```python
from build123d import *
from build123d.topology import SkipClean

# Parameters (mm, degrees)
ESBO_O1_R                = 2
RESSALTO_EXTRUS_O1_DEPTH = 19
CORTE_EXTRUS_O1_DEPTH    = 18
ESBO_O3_R                = 2.5
RESSALTO_EXTRUS_O2_DEPTH = 7


with BuildPart() as part:
    # Esboço1 → Ressalto-extrusão1 (new body)
    with BuildSketch(Plane.XY):
        with BuildLine():
            Line((19, 3.5), (13.555441712, 3.5))
            ThreePointArc((13.555441712, 3.5), (0, 14), (-13.555441712, 3.5))
            Line((-13.555441712, 3.5), (-19, 3.5))
            ThreePointArc((-19, 3.5), (-22.5, 0), (-19, -3.5))
            Line((-19, -3.5), (-13.555441712, -3.5))
            ThreePointArc((-13.555441712, -3.5), (-11.320120282, -8.237407166), (-7.5, -11.821590418))
            Line((-7.5, -11.821590418), (-7.5, -14))
            Line((-7.5, -14), (-7.5, -17))
            Line((-7.5, -17), (7.5, -17))
            Line((7.5, -17), (7.5, -14))
            Line((7.5, -14), (7.5, -11.821590418))
            ThreePointArc((7.5, -11.821590418), (11.320120282, -8.237407166), (13.555441712, -3.5))
            Line((13.555441712, -3.5), (19, -3.5))
            ThreePointArc((19, -3.5), (22.5, 0), (19, 3.5))
        make_face()
        with Locations((19, 0)):
            Circle(ESBO_O1_R, mode=Mode.SUBTRACT)
        with Locations(Location((-19, 0, 0), (0, 0, 180))):
            Circle(ESBO_O1_R, mode=Mode.SUBTRACT)
    extrude(amount=RESSALTO_EXTRUS_O1_DEPTH)

    # Esboço2 → Corte-extrusão1 (cut)
    with SkipClean():  # the faces are left unmerged after this step: merging them gives an invalid solid
        with BuildSketch(Plane(origin=(0, 0, 0), x_dir=(-1, 0, 0), z_dir=(0, 0, -1))):
            with BuildLine():
                Line((13.555441712, 3.5), (23.80699558, 3.5))
                Line((23.80699558, 3.5), (23.80699558, -3.5))
                Line((23.80699558, -3.5), (13.555441712, -3.5))
                ThreePointArc((13.555441712, -3.5), (14, 0), (13.555441712, 3.5))
            make_face()
            with BuildLine():
                Line((-13.555441712, 3.5), (-24.760546325, 3.5))
                Line((-24.760546325, 3.5), (-24.760546325, -3.5))
                Line((-24.760546325, -3.5), (-13.555441712, -3.5))
                ThreePointArc((-13.555441712, -3.5), (-14, 0), (-13.555441712, 3.5))
            make_face()
        extrude(amount=-CORTE_EXTRUS_O1_DEPTH, mode=Mode.SUBTRACT)

    # Esboço3 → Ressalto-extrusão2 (add)
    with SkipClean():  # the faces are left unmerged after this step: merging them gives an invalid solid
        with BuildSketch(Plane.XY.offset(19)):
            with Locations((0, 6.5)):
                Circle(ESBO_O3_R)
        extrude(amount=RESSALTO_EXTRUS_O2_DEPTH)


solid = part.part
```
Geometry: final body of the model. Coordinates: model frame, mm. A direction names the side the tool comes from. Coordinates: 2 decimals unless noted, no trailing zeros. Loops run counter-clockwise (first coordinate to the right, second up) from the corner with the lowest first, then second, coordinate; pieces in that order, holes last. Notation, with made-up numbers: (64, 6) -> (91, 6) arc R15 cw to (91, 33) -> close; hole circle Ø6 at (-37.5, 65). An arc over 180 degrees is marked (long way). Use a Markdown table: item, result. Add a question column.
(1) Section query D-D, the plane x = 18. Return loops of the section in (y, z), plus the area to 3 significant figures.
(2) Section query A-A, the plane y = 0. Return loops of the section in (x, z).
(3) Mould query, pull axis Y, two halves, no side actions, for faces 6 (the cylindrical face through (17.4, -1.2, 18.5)), 7 (the flat face through (0, -1, 19)), 8 (the cylindrical face through (-17.4, 1.2, 18.5)), 9 (the flat face through (-16.2, 3.5, 18.5)). Classes: pulls with the +Y half, pulls with the -Y half, needs draft (parallel to the pull), parting line crosses it, or undercut.
(4) Section query B-B, the plane z = 14.5. Return loops of the section in (x, y).
(5) Line query: line 1 along Y through (x, z) = (-19, 18.45); line 2 along Z through (x, y) = (2, 11.5); line 3 along Z through (x, y) = (-14.5, 2.5). Output: solid intervals per line, ascending.
(6) Section query C-C, the plane x = 0. Return loops of the section in (y, z).
(7) Access query for faces 1 (the flat face through (16.3, 3.5, 18.5)), 2 (the cylindrical face through (0, 9, 22)), 3 (the flat face through (-7.5, -14, 9)), 4 (the cylindrical face through (-22.5, 0.1, 18.5)), 5 (the flat face through (7.5, -14, 9)). Directions: +Z, -Z, +X, -X, +Y, -Y. A direction counts if a zero-diameter tool reaches every point of the face in a straight line with its end or side. Return the directions, or none.
(8) Pin query (flat end, axial travel): pin 1 Ø4 at (x, z) = (6, 18.5) entering from +Y; pin 2 Ø3.5 at (x, y) = (-19, 0) entering from -Z; pin 3 Ø0.5 at (x, z) = (-16.5, 18.5) entering from -Y; pin 4 Ø10 at (y, z) = (5, 6) entering from -X. Return the tip coordinate at first contact, or that it passes through.
Answer:
| question | item | result |
|---|---|---|
| 1 | outline | (-3.5, 18) -> (-1.73, 18) -> (-1.73, 19) -> (-3.5, 19) -> close; (1.73, 18) -> (3.5, 18) -> (3.5, 19) -> (1.73, 19) -> close |
| 1 | area | 3.54 mm^2 |
| 2 | outline | (-22.5, 18) -> (-21, 18) -> (-21, 19) -> (-22.5, 19) -> close; (-17, 18) -> (-14, 18) -> (-14, 0) -> (14, 0) -> (14, 18) -> (17, 18) -> (17, 19) -> (-17, 19) -> close; (21, 18) -> (22.5, 18) -> (22.5, 19) -> (21, 19) -> close |
| 3 | face 6 | undercut |
| 3 | face 7 | needs draft |
| 3 | face 8 | undercut |
| 3 | face 9 | pulls with the +Y half |
| 4 | outline | (-7.5, -17) -> (7.5, -17) -> (7.5, -11.82) arc R14 ccw (long way) to (-7.5, -11.82) -> close |
| 5 | line 1 | y = -3.5 to -2, 2 to 3.5 |
| 5 | line 2 | z = 0 to 19 |
| 5 | line 3 | z = 18 to 19 |
| 6 | outline | (-17, 0) -> (14, 0) -> (14, 19) -> (9, 19) -> (9, 26) -> (4, 26) -> (4, 19) -> (-17, 19) -> close |
| 7 | face 1 | +Z, -Z, +X, +Y |
| 7 | face 2 | +Z |
| 7 | face 3 | +Z, -Z, -X, -Y |
| 7 | face 4 | +Z, -Z, -X |
| 7 | face 5 | +Z, -Z, +X, -Y |
| 8 | pin 1 | stops at y = 13.42 |
| 8 | pin 2 | passes through |
| 8 | pin 3 | stops at y = -3.5 |
| 8 | pin 4 | stops at x = -14 |
